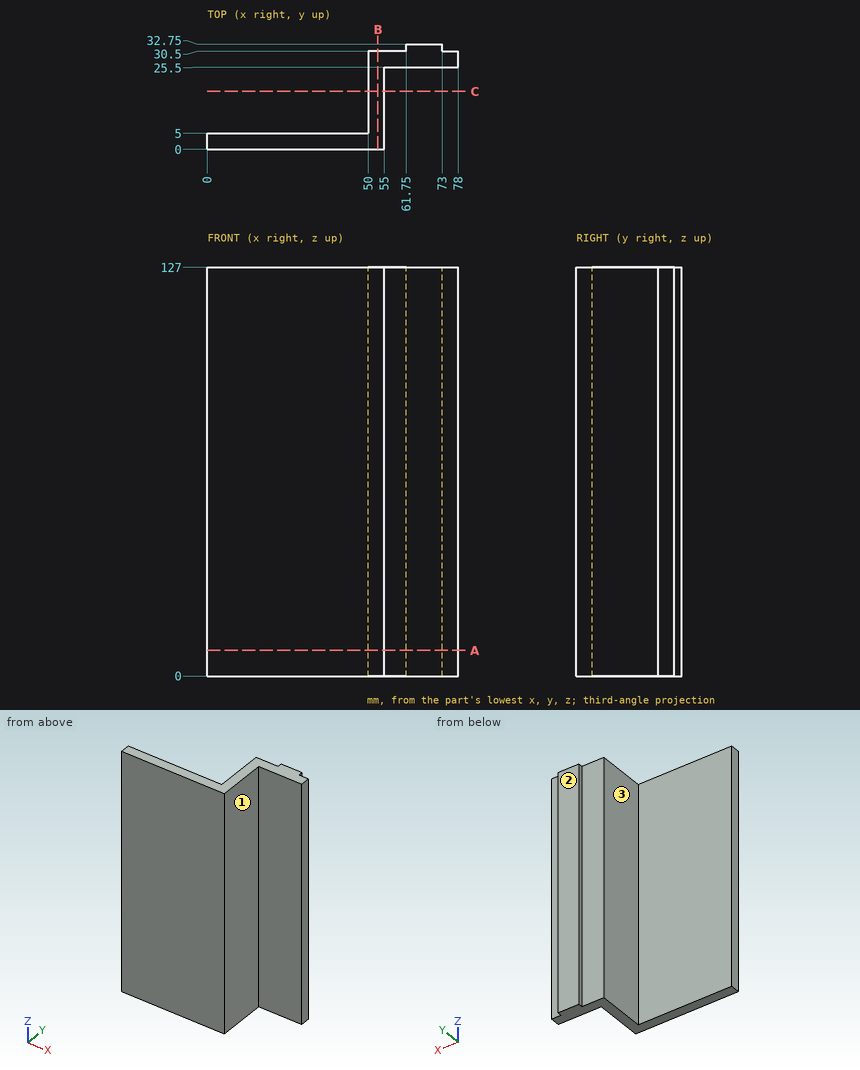
Verification items for this drawing (mm, ordinates from the low corner). A direction names the side the tool comes from. Give positions to 0.01 mm unless a question says otherwise; leave off trailing zeros. Loops run counter-clockwise (first coordinate to the right, second up) from the corner with the lowest first, then second, coordinate; pieces in that order, holes last. Notation, with made-up numbers: M 52.5,-37 L 81.5,-37 A8 ccw 81.5,-24 Z; hole C -1.5,49.5 d9. An arc over 180 degrees is marked long. Answer as CSV lines item,"result".
Item 1: Cross-section at B-B on x = 53. Record the cut outline in (y, z), and give its area (3 significant figures).
Values:
outline,"M 0,0 L 30.5,0 L 30.5,127 L 0,127 Z"
area,"3,870 mm²"
Item 2: Cross-section at A-A on z = 8. Record the cut outline in (x, y), and give its area (3 significant figures).
Values:
outline,"M 0,0 L 55,0 L 55,25.5 L 78,25.5 L 78,30.5 L 73,30.5 L 73,32.75 L 61.75,32.75 L 61.75,30.5 L 50,30.5 L 50,5 L 0,5 Z"
area,"543 mm²"
Item 3: Depth check by flat-ended pin: P1, Ø11.5, axis at x = 70, z = 92, coming from the -Y side; P2, Ø7.5, axis at y = 19, z = 33.5, coming from the -X side; P3, Ø3, axis at y = 17.5, z = 42.5, coming from the +X side. Enter the tip coordinate at first touch or a pass-through.
Values:
P1,"stops at y = 25.5"
P2,"stops at x = 50"
P3,"stops at x = 55"
Item 4: Material ranges on line 1 (Y direction, x = 51.5, z = 31); line 2 (X direction, y = 17, z = 51); line 3 (Y direction, x = 25.5, z = 47.5), recorded low to high.
Values:
line 1,"y = 0 to 30.5"
line 2,"x = 50 to 55"
line 3,"y = 0 to 5"
Item 5: Access from +Z, -Z, +X, -X, +Y, -Y to the whole of each face (thin tool, end or side, straight path). Record for the marked faces 1, 2 and 3.
Values:
face 1,"+Z, -Z, +X, -Y"
face 2,"+Z, -Z, +X, -X, +Y"
face 3,"+Z, -Z, -X, +Y"
Item 6: Cross-section at C-C on y = 18. Record the cut outline in (x, z).
Values:
outline,"M 50,0 L 55,0 L 55,127 L 50,127 Z"
